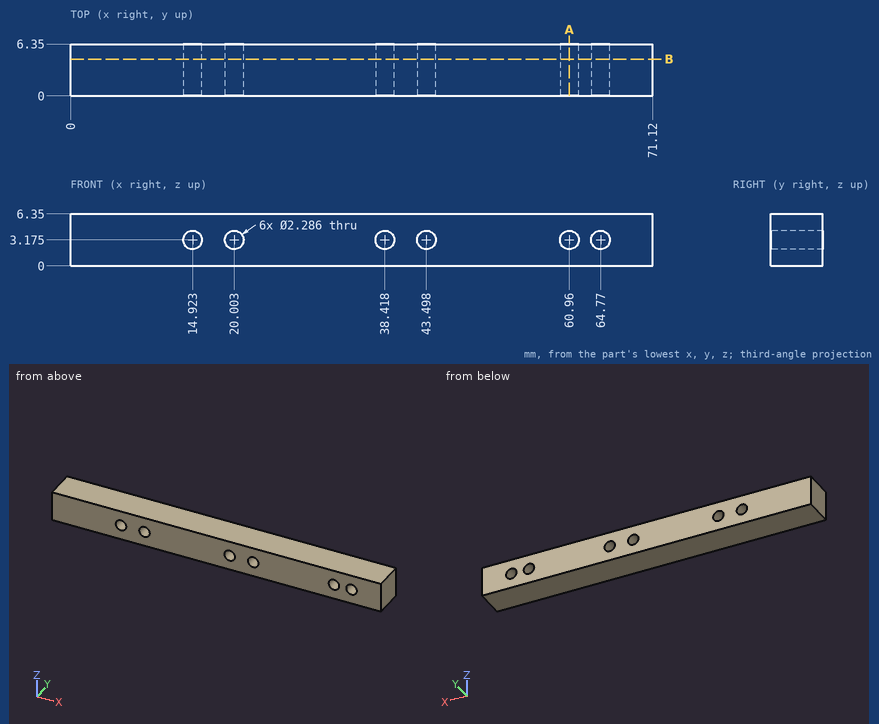
Can you work these out from the drawing? Everything is in mm from the part's minimum corner. Round coordinates to 2 decimals unless told otherwise and drop trailing zeros. Order: outer loops, then holes, each group sorted by start corner. A loop starts at its lowest first (then second) coordinate and runs counter-clockwise, first axis right, second up. Notation, with made-up numbers: (88.5, 34.25) -> (137.5, 34.25) arc R12 cw to (137.5, 50.25) -> close; hole circle Ø10 at (62, 9). An arc over 180 degrees is marked (long way). Use CSV: the item, a comma, the result in double quotes.
1. I want a section at A-A on x = 60.96. List the corners of the cut face in (y, z) for me.
Recorded:
outline,"(0, 0) -> (6.35, 0) -> (6.35, 2.03) -> (0, 2.03) -> close; (0, 4.32) -> (6.35, 4.32) -> (6.35, 6.35) -> (0, 6.35) -> close"
2. I'm going to push flat-ended pins straight in: P1, Ø3.5, axis at x = 64.77, z = 3.175, coming from the +Y side; P2, Ø1.4, axis at x = 20, z = 3.18, coming from the +Y side. Where does each tip first touch, or does it pass through?
Recorded:
P1,"stops at y = 6.35"
P2,"passes through"
3. I want a section at B-B on y = 4.5. Give the number of separate pieces and of enclosed holes in the cut face, and give its area (3 significant figures).
Recorded:
separate pieces,"1"
enclosed holes,"6"
area,"427 mm2"
4. I need wall thicknesses on line 1 along Z through (x, y) = (61, 3.25); line 2 along Z through (x, y) = (19.5, 1.25). Which ranges of each line are inside material? Lowest first, please.
Recorded:
line 1,"z = 0 to 2.03, 4.32 to 6.35"
line 2,"z = 0 to 2.15, 4.2 to 6.35"
